Can you work these out from the model? Positions are in its coordinate system, mm. A direction names the side the tool comes from. Round coordinates to 2 decimals unless told otherwise and drop trailing zeros. Write each loop counter-clockwise with the first axis right and the second up, starting at its lowest first coordinate (ties: lowest second). Pieces come first, ordered by that corner, then holes.
Q1. If we section it at B-B (y = 99): Please give me the cut outline in (x, z) (3 decimals).
Q2. If we section it at A-A (x = 324.5): Please give me the cut outline in (y, z) (3 decimals), plus the area to 3 significant figures.
Q3. I'm going to push flat-ended pins straight in: pin 1 Ø5 at (x, y) = (-530.5, 146.5) entering from +Z (3 decimals); pin 2 Ø6.5 at (x, y) = (101.6, 38.1) entering from +Z; pin 3 Ø5 at (y, z) = (112, -530.5) entering from -X; pin 4 Ø11.5 at (x, z) = (381, -587.375) entering from -Y (3 decimals). Where does each tip first touch, or does it pass through?
Q4. Please list where these lines run through material, in increasing order: line 1 along X through (y, z) = (38, -533); line 2 along Z through (x, y) = (381, 147.25); line 3 along Y through (x, z) = (101, -533).
Q5. For faces 1 (the flat face through (583, 148, -583)), 2 (the flat face through (-7, 70, -536.575)), which set-ups out of +Z, -Z, +X, -X, +Y, -Y let a thin tool reach every point of the face, with its end or its side?
from build123d import *

# Parameters (mm, degrees)
SKETCH3_W                                        = 1073.15
SKETCH3_H                                        = 1073.15
BOSS_EXTRUDE1_DEPTH                              = 152.4
SKETCH4_OUTSIDE_W                                = 1380.21
SKETCH4_OUTSIDE_H                                = 1380.21
SKETCH4_OUTSIDE_W_2                              = 1073.15
SKETCH4_OUTSIDE_H_2                              = 1073.15
SKETCH4_OUTSIDE_W_3                              = 1054.1
SKETCH4_OUTSIDE_H_3                              = 1054.1
CUT_EXTRUDE3_DEPTH                               = 142.875
SKETCH5_W                                        = 1358.9
SKETCH5_H                                        = 1358.9
SKETCH5_W_2                                      = 1073.15
SKETCH5_H_2                                      = 1073.15
BOSS_EXTRUDE2_DEPTH                              = 9.525
SKETCH6_W                                        = 1054.1
SKETCH6_H                                        = 1054.1
CUT_EXTRUDE5_DEPTH                               = 9.525
SKETCH7_R                                        = 4.365625
SKETCH7_R_2                                      = 4.36499
CUT_EXTRUDE6_DEPTH                               = 9.525
SKETCH8_R                                        = 2.50063
CUT_EXTRUDE7_DEPTH                               = 1270
SKETCH9_R                                        = 2.50063
CUT_EXTRUDE8_DEPTH                               = 1270
SKETCH10_R                                       = 3.5687
CUT_EXTRUDE10_DEPTH                              = 1270
SKETCH11_W                                       = 1358.9
SKETCH11_H                                       = 1358.9
SKETCH11_W_2                                     = 1206.5
SKETCH11_H_2                                     = 1206.5
CUT_EXTRUDE11_DEPTH                              = 9.525
CUT_EXTRUDE12_DEPTH                              = 254
CUT_EXTRUDE13_DEPTH                              = 867.629612349
CSK_FOR_1_4_FLAT_HEAD_MACHINE_SCREW1_D           = 7.1374
CSK_FOR_1_4_FLAT_HEAD_MACHINE_SCREW1_CSINK_D     = 15.637764
CSK_FOR_1_4_FLAT_HEAD_MACHINE_SCREW1_CSINK_ANGLE = 82
CSK_FOR_1_4_FLAT_HEAD_MACHINE_SCREW2_D           = 7.1374
CSK_FOR_1_4_FLAT_HEAD_MACHINE_SCREW2_CSINK_D     = 15.637764
CSK_FOR_1_4_FLAT_HEAD_MACHINE_SCREW2_CSINK_ANGLE = 82
CSK_FOR_1_4_FLAT_HEAD_MACHINE_SCREW3_D           = 7.1374
CSK_FOR_1_4_FLAT_HEAD_MACHINE_SCREW3_CSINK_D     = 15.637764
CSK_FOR_1_4_FLAT_HEAD_MACHINE_SCREW3_CSINK_ANGLE = 82
CSK_FOR_1_4_FLAT_HEAD_MACHINE_SCREW5_D           = 7.1374
CSK_FOR_1_4_FLAT_HEAD_MACHINE_SCREW5_CSINK_D     = 15.5273756
CSK_FOR_1_4_FLAT_HEAD_MACHINE_SCREW5_CSINK_ANGLE = 82
BOSS_EXTRUDE3_DEPTH                              = 9.525


with BuildPart() as part:
    # Sketch3 → Boss-Extrude1 (new body)
    with BuildSketch(Plane(origin=(0, 0, 0), x_dir=(1, 0, 0), z_dir=(0, 1, 0))):
        Rectangle(SKETCH3_W, SKETCH3_H)
    extrude(amount=BOSS_EXTRUDE1_DEPTH)

    # Sketch4 outside → Cut-Extrude3 (cut)
    # profile 1 of 2: a face of its own
    with BuildSketch(Plane(origin=(0, 152.4, 0), x_dir=(1, 0, 0), z_dir=(0, 1, 0))):
        Rectangle(SKETCH4_OUTSIDE_W, SKETCH4_OUTSIDE_H)
        Rectangle(SKETCH4_OUTSIDE_W_2, SKETCH4_OUTSIDE_H_2, mode=Mode.SUBTRACT)
    # profile 2 of 2: a face of its own
    with BuildSketch(Plane(origin=(0, 152.4, 0), x_dir=(1, 0, 0), z_dir=(0, 1, 0))):
        Rectangle(SKETCH4_OUTSIDE_W_3, SKETCH4_OUTSIDE_H_3)
    extrude(amount=-CUT_EXTRUDE3_DEPTH, mode=Mode.SUBTRACT)

    # Sketch5 → Boss-Extrude2 (add)
    with BuildSketch(Plane(origin=(0, 152.4, 0), x_dir=(1, 0, 0), z_dir=(0, 1, 0))):
        Rectangle(SKETCH5_W, SKETCH5_H)
        Rectangle(SKETCH5_W_2, SKETCH5_H_2, mode=Mode.SUBTRACT)
    extrude(amount=-BOSS_EXTRUDE2_DEPTH)

    # Sketch6 → Cut-Extrude5 (cut)
    with BuildSketch(Plane(origin=(0, 9.525, 0), x_dir=(1, 0, 0), z_dir=(0, 1, 0))):
        Rectangle(SKETCH6_W, SKETCH6_H)
    extrude(amount=-CUT_EXTRUDE5_DEPTH, mode=Mode.SUBTRACT)

    # Sketch7 → Cut-Extrude6 (cut)
    with BuildSketch(Plane(origin=(0, 152.4, 0), x_dir=(1, 0, 0), z_dir=(0, 1, 0))):
        with Locations(Location((549.275, 38.1, 0), (0, 0, 270))):
            Circle(SKETCH7_R)
        with Locations(Location((587.375, -38.1, 0), (0, 0, 270))):
            Circle(SKETCH7_R)
        with Locations(Location((549.275, -38.1, 0), (0, 0, 270))):
            Circle(SKETCH7_R)
        with Locations(Location((587.375, 38.1, 0), (0, 0, 270))):
            Circle(SKETCH7_R)
        with Locations(Location((549.275, 419.1, 0), (0, 0, 270))):
            Circle(SKETCH7_R)
        with Locations(Location((549.275, 342.9, 0), (0, 0, 270))):
            Circle(SKETCH7_R)
        with Locations(Location((587.375, 342.9, 0), (0, 0, 270))):
            Circle(SKETCH7_R)
        with Locations(Location((587.375, 419.1, 0), (0, 0, 270))):
            Circle(SKETCH7_R)
        with Locations(Location((587.375, -419.1, 0), (0, 0, 270))):
            Circle(SKETCH7_R)
        with Locations(Location((549.275, -419.1, 0), (0, 0, 270))):
            Circle(SKETCH7_R)
        with Locations(Location((587.375, -342.9, 0), (0, 0, 270))):
            Circle(SKETCH7_R)
        with Locations(Location((549.275, -342.9, 0), (0, 0, 270))):
            Circle(SKETCH7_R)
        with Locations(Location((-549.275, -38.1, 0), (0, 0, 270))):
            Circle(SKETCH7_R)
        with Locations(Location((-549.275, 419.1, 0), (0, 0, 270))):
            Circle(SKETCH7_R)
        with Locations(Location((-549.275, 342.9, 0), (0, 0, 270))):
            Circle(SKETCH7_R)
        with Locations(Location((-549.275, -342.9, 0), (0, 0, 270))):
            Circle(SKETCH7_R)
        with Locations(Location((-549.275, 38.1, 0), (0, 0, 270))):
            Circle(SKETCH7_R)
        with Locations(Location((-549.275, -419.1, 0), (0, 0, 270))):
            Circle(SKETCH7_R)
        with Locations(Location((-342.9, -549.275, 0), (0, 0, 270))):
            Circle(SKETCH7_R)
        with Locations(Location((-38.1, -549.275, 0), (0, 0, 270))):
            Circle(SKETCH7_R)
        with Locations(Location((419.1, -549.275, 0), (0, 0, 270))):
            Circle(SKETCH7_R)
        with Locations(Location((342.9, -549.275, 0), (0, 0, 270))):
            Circle(SKETCH7_R)
        with Locations(Location((38.1, -549.275, 0), (0, 0, 270))):
            Circle(SKETCH7_R)
        with Locations(Location((-419.1, -549.275, 0), (0, 0, 270))):
            Circle(SKETCH7_R)
        with Locations(Location((-584.2, -342.9, 0), (0, 0, 270))):
            Circle(SKETCH7_R)
        with Locations(Location((-584.2, -419.1, 0), (0, 0, 270))):
            Circle(SKETCH7_R)
        with Locations(Location((-584.2, 342.9, 0), (0, 0, 270))):
            Circle(SKETCH7_R)
        with Locations(Location((-584.2, -38.1, 0), (0, 0, 270))):
            Circle(SKETCH7_R)
        with Locations(Location((-584.2, 419.1, 0), (0, 0, 270))):
            Circle(SKETCH7_R)
        with Locations(Location((-584.2, 38.1, 0), (0, 0, 270))):
            Circle(SKETCH7_R)
        with Locations(Location((-342.9, -584.2, 0), (0, 0, 270))):
            Circle(SKETCH7_R)
        with Locations(Location((-419.1, -584.2, 0), (0, 0, 270))):
            Circle(SKETCH7_R)
        with Locations(Location((38.1, -584.2, 0), (0, 0, 270))):
            Circle(SKETCH7_R)
        with Locations(Location((419.1, -584.2, 0), (0, 0, 270))):
            Circle(SKETCH7_R)
        with Locations(Location((-38.1, -584.2, 0), (0, 0, 270))):
            Circle(SKETCH7_R)
        with Locations(Location((342.9, -584.2, 0), (0, 0, 270))):
            Circle(SKETCH7_R)
        with Locations(Location((-381, 587.375, 0), (0, 0, 270))):
            Circle(SKETCH7_R_2)
        with Locations(Location((-381, 549.275, 0), (0, 0, 270))):
            Circle(SKETCH7_R_2)
        with Locations(Location((0, 587.375, 0), (0, 0, 270))):
            Circle(SKETCH7_R_2)
        with Locations(Location((0, 549.275, 0), (0, 0, 270))):
            Circle(SKETCH7_R_2)
        with Locations(Location((381, 587.375, 0), (0, 0, 270))):
            Circle(SKETCH7_R_2)
        with Locations(Location((381, 549.275, 0), (0, 0, 270))):
            Circle(SKETCH7_R_2)
    extrude(amount=-CUT_EXTRUDE6_DEPTH, mode=Mode.SUBTRACT)

    # Sketch8 → Cut-Extrude7 (cut)
    with BuildSketch(Plane.ZY.offset(536.575)):
        with Locations((371.475, 38.1)):
            Circle(SKETCH8_R)
    extrude(amount=-CUT_EXTRUDE7_DEPTH, mode=Mode.SUBTRACT)

    # Sketch9 → Cut-Extrude8 (cut)
    with BuildSketch(Plane.ZY.offset(536.575)):
        with Locations((-371.475, 38.1)):
            Circle(SKETCH9_R)
        with Locations((-222.885, 38.1)):
            Circle(SKETCH9_R)
        with Locations((-74.295, 38.1)):
            Circle(SKETCH9_R)
        with Locations((74.295, 38.1)):
            Circle(SKETCH9_R)
        with Locations((222.885, 38.1)):
            Circle(SKETCH9_R)
    extrude(amount=-CUT_EXTRUDE8_DEPTH, mode=Mode.SUBTRACT)

    # Sketch10 → Cut-Extrude10 (cut)
    with BuildSketch(Plane.XY.offset(536.575)):
        with Locations((-304.8, 38.1)):
            Circle(SKETCH10_R)
        with Locations((-101.6, 38.1)):
            Circle(SKETCH10_R)
        with Locations((101.6, 38.1)):
            Circle(SKETCH10_R)
        with Locations((304.8, 38.1)):
            Circle(SKETCH10_R)
    extrude(amount=-CUT_EXTRUDE10_DEPTH, mode=Mode.SUBTRACT)

    # Sketch11 → Cut-Extrude11 (cut)
    with BuildSketch(Plane(origin=(0, 152.4, 0), x_dir=(1, 0, 0), z_dir=(0, 1, 0))):
        Rectangle(SKETCH11_W, SKETCH11_H)
        Rectangle(SKETCH11_W_2, SKETCH11_H_2, mode=Mode.SUBTRACT)
    extrude(amount=-CUT_EXTRUDE11_DEPTH, mode=Mode.SUBTRACT)

    # Sketch12 → Cut-Extrude12 (cut)
    with BuildSketch(Plane(origin=(0, 152.4, 0), x_dir=(1, 0, 0), z_dir=(0, 1, 0))):
        Polygon((-527.05, 527.05), (-527.05, -527.05), (527.05, -527.05), (527.05, 527.05), (603.25, 603.25), (603.25, -603.25), (-603.25, -603.25), (-603.25, 603.25), align=None)
    extrude(amount=-CUT_EXTRUDE12_DEPTH, mode=Mode.SUBTRACT)

    # Sketch14 → Cut-Extrude13 (cut, through all)
    with BuildSketch(Plane.XZ):
        Polygon((-527.05, -527.05), (-536.575, -536.575), (-527.05, -536.575), align=None)
        Polygon((536.575, -536.575), (527.05, -536.575), (527.05, -527.05), align=None)
    extrude(amount=-CUT_EXTRUDE13_DEPTH, mode=Mode.SUBTRACT)

    # CSK for 1/4 Flat Head Machine Screw1 (through all)
    with Locations(Plane(origin=(-304.8, 38.1, -527.05), x_dir=(1, 0, 0), z_dir=(0, 0, 1))):
        with Locations((0, 0)):
            CounterSinkHole(CSK_FOR_1_4_FLAT_HEAD_MACHINE_SCREW1_D / 2, CSK_FOR_1_4_FLAT_HEAD_MACHINE_SCREW1_CSINK_D / 2, counter_sink_angle=CSK_FOR_1_4_FLAT_HEAD_MACHINE_SCREW1_CSINK_ANGLE)

    # CSK for 1/4 Flat Head Machine Screw2 (through all)
    with Locations(Plane(origin=(-101.6, 38.1, -527.05), x_dir=(1, 0, 0), z_dir=(0, 0, 1))):
        with Locations((0, 0)):
            CounterSinkHole(CSK_FOR_1_4_FLAT_HEAD_MACHINE_SCREW2_D / 2, CSK_FOR_1_4_FLAT_HEAD_MACHINE_SCREW2_CSINK_D / 2, counter_sink_angle=CSK_FOR_1_4_FLAT_HEAD_MACHINE_SCREW2_CSINK_ANGLE)

    # CSK for 1/4 Flat Head Machine Screw3 (through all)
    with Locations(Plane(origin=(101.6, 38.1, -527.05), x_dir=(1, 0, 0), z_dir=(0, 0, 1))):
        with Locations((0, 0)):
            CounterSinkHole(CSK_FOR_1_4_FLAT_HEAD_MACHINE_SCREW3_D / 2, CSK_FOR_1_4_FLAT_HEAD_MACHINE_SCREW3_CSINK_D / 2, counter_sink_angle=CSK_FOR_1_4_FLAT_HEAD_MACHINE_SCREW3_CSINK_ANGLE)

    # CSK for 1/4 Flat Head Machine Screw5 (through all)
    with Locations(Plane(origin=(304.8, 38.1, -527.05), x_dir=(1, 0, 0), z_dir=(0, 0, 1))):
        with Locations((0, 0)):
            CounterSinkHole(CSK_FOR_1_4_FLAT_HEAD_MACHINE_SCREW5_D / 2, CSK_FOR_1_4_FLAT_HEAD_MACHINE_SCREW5_CSINK_D / 2, counter_sink_angle=CSK_FOR_1_4_FLAT_HEAD_MACHINE_SCREW5_CSINK_ANGLE)

    # Sketch22 → Boss-Extrude3 (add)
    with BuildSketch(Plane(origin=(0, 152.4, 0), x_dir=(1, 0, 0), z_dir=(0, 1, 0))):
        Polygon((603.25, 603.25), (-603.25, 603.25), (-628.65, 628.65), (628.65, 628.65), align=None)
    extrude(amount=-BOSS_EXTRUDE3_DEPTH)


solid = part.part
A:
1. outline: (-527.05, -536.575) - (527.05, -536.575) - (527.05, -527.05) - (-527.05, -527.05) - close
2. outline: (0, -536.575) - (142.875, -536.575) - (142.875, -628.65) - (152.4, -628.65) - (152.4, -527.05) - (0, -527.05) - close
2. area: 2,330 mm2
3. pin 1: stops at z = -536.575
3. pin 2: passes through
3. pin 3: stops at x = -527.05
3. pin 4: stops at y = 142.875
4. line 1: x = -527.05 to -308.37, -301.23 to -105.17, -98.03 to 98.03, 105.17 to 301.23, 308.37 to 527.05
4. line 2: z = -628.65 to -591.74, -583.01 to -553.64, -544.91 to -527.05
4. line 3: y = 0 to 34.58, 41.62 to 152.4
5. face 1: +Z, +X, +Y, -Y
5. face 2: -Z, +X, -X, -Y
